Input: part model. Units: mm. Frame: model coordinates. Face numbers are marked on the shaded views. A direction names the side the tool comes from. Coordinates: 2 decimals unless noted, no trailing zeros. Loops run counter-clockwise (first coordinate to the right, second up) from the corner with the lowest first, then second, coordinate; pieces in that order, holes last. Notation, with made-up numbers: (15, 44.5) - (23, 44.5) arc R23 cw to (23, 70.5) - close; hole circle Ø7 at (26, 9.25). An arc over 180 degrees is marked (long way). Answer as CSV lines item,"result". Start each with the question number.
```python
from build123d import *


with BuildPart() as part:
    # Sketch1 → Revolve1 (revolve)
    with BuildSketch(Plane.XY, mode=Mode.PRIVATE) as revolve1_sk:
        with BuildLine():
            Line((0, 0), (0, 4))
            Line((0, 4), (5.665073225, 4))
            ThreePointArc((5.665073225, 4), (5.975896248, 3.689038292), (5.975798184, 3.249370092))
            add(Edge.make_bspline(
                [(0, 0), (4.05719651, 0.732493998), (5.691820154, 2.564218754), (5.975798184, 3.249370092)],
                knots=[0, 0, 0, 0, 1, 1, 1, 1], degree=3))
        make_face()
        Polygon((0, 13), (0, 4), (3.5, 4), (3.5, 6.5), (2.5, 6.5), (2.5, 13), align=None)
    revolve(revolve1_sk.sketch.rotate(Axis((0, 0, 0), (0, 1, 0)), 90), axis=Axis((0, 0, 0), (0, 1, 0)))


solid = part.part
```
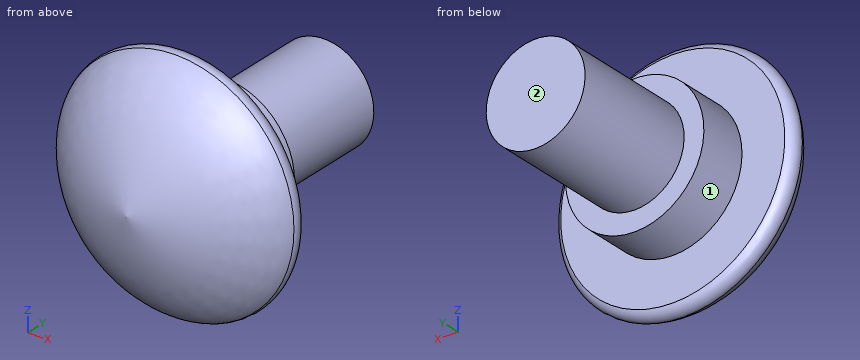
Item 1: Set-up query: the marked faces 1 and 2. Return all of +Z, -Z, +X, -X, +Y, -Y with unobstructed straight access to the full face (end or side cutting, diameter ignored); none if empty.
Item 2: Section query A-A, the plane y = 10.25. Output: boundary loops of the cut face in (x, z), and give its area (3 significant figures).
Item 3: Material intervals for probe 1 along Y at (x, z) = (-3, 2.75); probe 2 along X at (y, z) = (9.75, -1.25); probe 3 along Z at (x, y) = (1.75, 1.5), sorted ascending.
Item 4: Contact query for flat-ended pins moving along their axis: P1, Ø6, axis at y = 2.5, z = 5, coming from the -X side; P2, Ø6, axis at x = 1.5, y = 10.5, coming from the -Z side; P3, Ø1.5, axis at y = 4, z = -3, coming from the -X side. Output: stop coordinate, or through.
Response values:
1,face 1,"+Y"
1,face 2,"+Z, -Z, +X, -X, +Y"
2,outline,"circle Ø5 at (0, 0)"
2,area,"19.6 mm²"
3,probe 1,"y = 1.43 to 4"
3,probe 2,"x = -2.17 to 2.17"
3,probe 3,"z = -3.8 to 3.8"
4,P1,"stops at x = -5.62"
4,P2,"stops at z = -2.5"
4,P3,"stops at x = -5.52"
